Job drawing, mm, ordinate dimensions from the low corner. One solid piece. Round coordinates to 2 decimals unless told otherwise and drop trailing zeros. Loops run counter-clockwise (first coordinate to the right, second up) from the corner with the lowest first, then second, coordinate; pieces in that order, holes last. Notation, with made-up numbers: M 4.5,48 L 41.5,48 A10 cw 41.5,57 Z; hole C 45.25,-18 d9. An arc over 180 degrees is marked long. One line per item, written item: value.
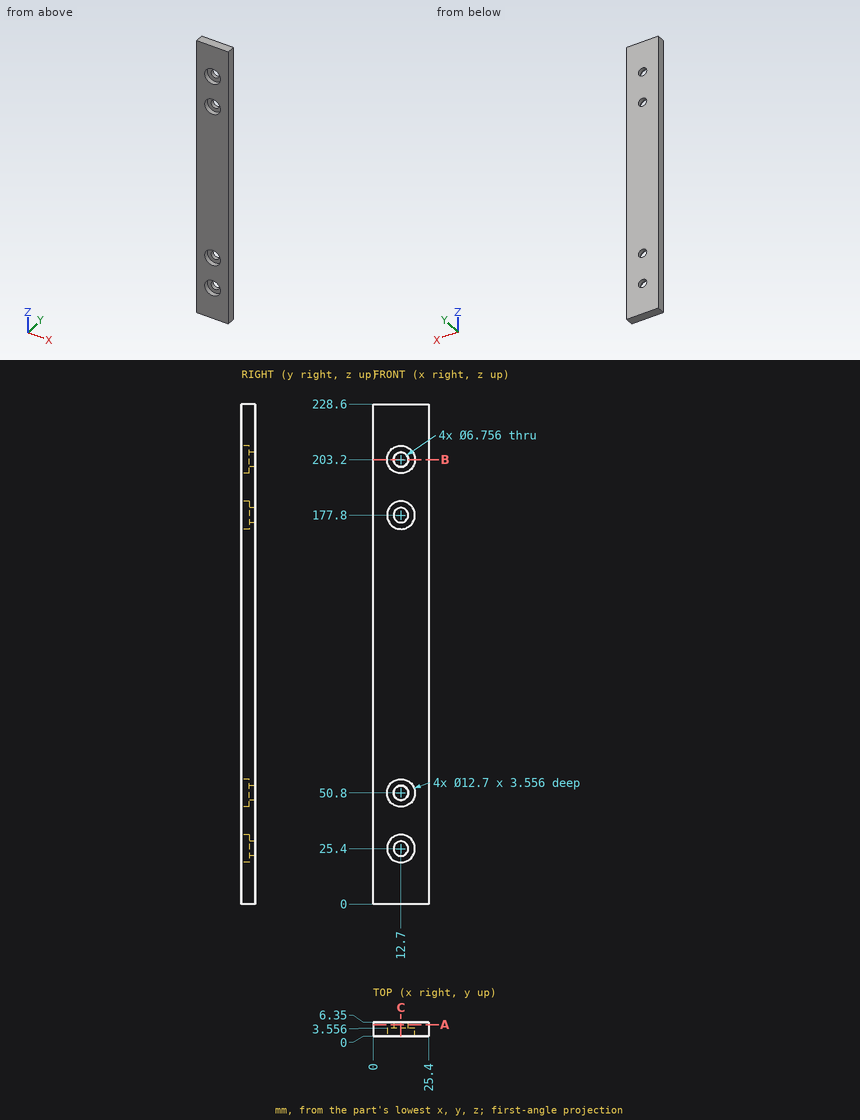
Item 1: Wall check: line 1 along Z through (x, y) = (12.7, 2.6); line 2 along Z through (x, y) = (12.7, 4.5); line 3 along X through (y, z) = (5.15, 177.8). Give the ranges that are in metal, low to high.
Check values:
line 1: z = 0 to 19.05, 31.75 to 44.45, 57.15 to 171.45, 184.15 to 196.85, 209.55 to 228.6
line 2: z = 0 to 22.02, 28.78 to 47.42, 54.18 to 174.42, 181.18 to 199.82, 206.58 to 228.6
line 3: x = 0 to 9.32, 16.08 to 25.4
Item 2: Drop a flat-ended pin along its axis: P1, Ø8, axis at x = 12.7, z = 177.8, coming from the -Y side. Give the stop position or say it passes through.
Check values:
P1: stops at y = 3.56
Item 3: Slice it at C-C, the plane x = 12.7. Give the number of separate pieces and of enclosed holes in the cut face, and give its area (3 significant figures).
Check values:
separate pieces: 5
enclosed holes: 0
area: 1,200 mm2
Item 4: Slice it at A-A, the plane y = 5.25. Give the cut face in (x, z).
Check values:
outline: M 0,0 L 25.4,0 L 25.4,228.6 L 0,228.6 Z; hole C 12.7,25.4 d6.76; hole C 12.7,50.8 d6.76; hole C 12.7,177.8 d6.76; hole C 12.7,203.2 d6.76
Item 5: Slice it at B-B, the plane z = 203.2. Give the cut face in (x, y).
Check values:
outline: M 0,0 L 6.35,0 L 6.35,3.56 L 9.32,3.56 L 9.32,6.35 L 0,6.35 Z; M 16.08,3.56 L 19.05,3.56 L 19.05,0 L 25.4,0 L 25.4,6.35 L 16.08,6.35 Z
